from build123d import *

# Parameters (mm, degrees)
SKETCH1_R           = 23.8125
SKETCH1_R_2         = 20.6375
BOSS_EXTRUDE1_DEPTH = 8.89
BOSS_EXTRUDE2_START = -8.89
BOSS_EXTRUDE2_DEPTH = 8.89
FILLET1_R           = 25.4
CIRPATTERN1_DEPTH   = 8.89
SKETCH3_R           = 2.2225
CUT_EXTRUDE1_DEPTH  = 41.553113931
CIRPATTERN2_COUNT   = 6


# Read off the part's stored shape, not the designer's step: CirPattern1
with BuildPart() as part:
    # Sketch1 → Boss-Extrude1 (new body)
    with BuildSketch(Plane(origin=(0, 0, 0), x_dir=(1, 0, 0), z_dir=(0, 1, 0))):
        with Locations(Location((0, 0, 0), (0, 0, 270))):
            Circle(SKETCH1_R)
        with Locations(Location((0, 0, 0), (0, 0, 270))):
            Circle(SKETCH1_R_2, mode=Mode.SUBTRACT)
    extrude(amount=BOSS_EXTRUDE1_DEPTH)

    # Sketch2 → Boss-Extrude2 (add)
    with BuildSketch(Plane(origin=(0, 8.89, 0), x_dir=(1, 0, 0), z_dir=(0, 1, 0)).offset(BOSS_EXTRUDE2_START)):
        with BuildLine():
            ThreePointArc((-23.1267, 5.673702791), (-29.5275, 0), (-23.1267, -5.673702791))
            ThreePointArc((-23.1267, -5.673702791), (-23.8125, 0), (-23.1267, 5.673702791))
        make_face()
    extrude(amount=BOSS_EXTRUDE2_DEPTH)

    # Fillet1
    fillet1_edges = [part.edges().sort_by_distance(p)[0] for p in [
        (-23.1267, 4.445, -5.673702791),
        (-23.1267, 4.445, 5.673702791),
    ]]
    fillet(fillet1_edges, radius=FILLET1_R)

    # CirPattern1 outline → CirPattern1 (add)
    with BuildSketch(Plane(origin=(0, 0, 0), x_dir=(1, 0, 0), z_dir=(0, 1, 0))):
        with BuildLine():
            ThreePointArc((-20.530983871, -12.062912482), (-18.612348128, -16.535370154), (-17.581908256, -21.29165383))
            ThreePointArc((-17.581908256, -21.29165383), (-14.764885819, -25.570909171), (-9.650569001, -25.873242043))
            ThreePointArc((-9.650569001, -25.873242043), (-4.837563965, -24.35161844), (0.181296717, -23.811809838))
            ThreePointArc((0.181296717, -23.811809838), (-11.748897356, -20.712280588), (-20.530983871, -12.062912482))
        make_face()
        with BuildLine():
            ThreePointArc((-20.530983871, 12.062912482), (-11.90625, 20.622229928), (-0.181296717, 23.811809838))
            ThreePointArc((-0.181296717, 23.811809838), (-5.01387655, 24.38645138), (-9.648158978, 25.872206112))
            ThreePointArc((-9.648158978, 25.872206112), (-14.76375, 25.57156511), (-17.581908256, 21.29165383))
            ThreePointArc((-17.581908256, 21.29165383), (-18.612348128, 16.535370154), (-20.530983871, 12.062912482))
        make_face()
        with BuildLine():
            ThreePointArc((-0.181296717, 23.811809838), (11.748897356, 20.712280588), (20.530983871, 12.062912482))
            ThreePointArc((20.530983871, 12.062912482), (18.612348128, 16.535370154), (17.581908256, 21.29165383))
            ThreePointArc((17.581908256, 21.29165383), (14.764885819, 25.570909171), (9.650569001, 25.873242043))
            ThreePointArc((9.650569001, 25.873242043), (4.837563965, 24.35161844), (-0.181296717, 23.811809838))
        make_face()
        with BuildLine():
            ThreePointArc((20.530983871, 12.062912482), (23.811809838, 0.181296717), (20.712280588, -11.748897356))
            ThreePointArc((20.712280588, -11.748897356), (23.626224678, -7.851081226), (27.230067234, -4.580552281))
            ThreePointArc((27.230067234, -4.580552281), (29.527499849, -0.001311618), (27.232169388, 4.578983105))
            ThreePointArc((27.232169388, 4.578983105), (23.507902174, 7.986355934), (20.530983871, 12.062912482))
        make_face()
        with BuildLine():
            ThreePointArc((20.712280588, -11.748897356), (12.062912482, -20.530983871), (0.181296717, -23.811809838))
            ThreePointArc((0.181296717, -23.811809838), (5.01387655, -24.38645138), (9.648158978, -25.872206112))
            ThreePointArc((9.648158978, -25.872206112), (14.762614031, -25.572220789), (17.581600387, -21.294258937))
            ThreePointArc((17.581600387, -21.294258937), (18.67033821, -16.365262506), (20.712280588, -11.748897356))
        make_face()
    extrude(amount=CIRPATTERN1_DEPTH)

    # Sketch3 → Cut-Extrude1 (cut, symmetric)
    with BuildSketch(Plane(origin=(0, 8.89, 0), x_dir=(1, 0, 0), z_dir=(0, 1, 0))):
        with Locations(Location((-25.0825, 0, 0), (0, 0, 270))):
            Circle(SKETCH3_R)
    cut_extrude1 = extrude(amount=CUT_EXTRUDE1_DEPTH, both=True, mode=Mode.SUBTRACT)

    # CirPattern2: Cut-Extrude1 ×6 about axis
    cirpattern2_axis = Axis((0, 0, 0), (0, 1, 0))
    for i in range(1, CIRPATTERN2_COUNT):
        add(cut_extrude1.rotate(cirpattern2_axis, i * 360 / CIRPATTERN2_COUNT), mode=Mode.SUBTRACT)


solid = part.part
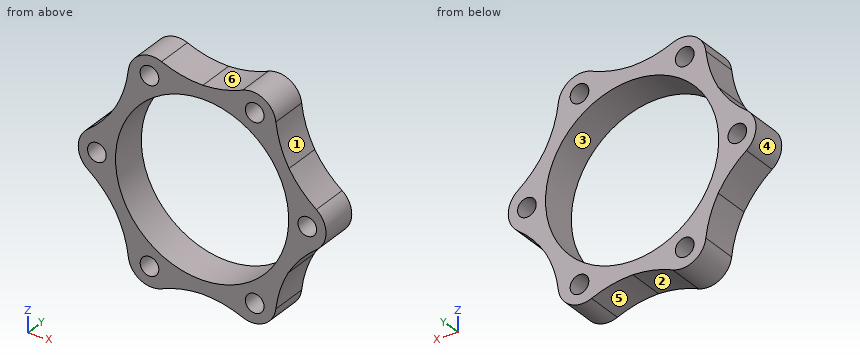
Read the model definition and answer for the solid it produces. Units are mm, in the model's axes. Face numbers are marked on the shaded views. A direction names the side the tool comes from. Round coordinates to 2 decimals unless told otherwise and drop trailing zeros. Write each loop counter-clockwise with the first axis right and the second up, starting at its lowest first coordinate (ties: lowest second). Pieces come first, ordered by that corner, then holes.
Q1. Find section D-D on x = 8. Determine the outline of the cut face in (y, z), and give its area (3 significant figures).
Values:
outline: (0, -25.23) - (8.89, -25.23) - (8.89, -19.02) - (0, -19.02) - close; (0, 19.02) - (8.89, 19.02) - (8.89, 25.23) - (0, 25.23) - close
area: 110 mm2
Q2. Find section A-A on z = 0. Determine the outline of the cut face in (x, y) (1 decimal).
Values:
outline: (-29.5, 0) - (-27.3, 0) - (-27.3, 8.9) - (-29.5, 8.9) - close; (-22.9, 0) - (-20.6, 0) - (-20.6, 8.9) - (-22.9, 8.9) - close; (20.6, 0) - (22.9, 0) - (22.9, 8.9) - (20.6, 8.9) - close; (27.3, 0) - (29.5, 0) - (29.5, 8.9) - (27.3, 8.9) - close
Q3. Straight lines are drawn through the part: line 1 (X direction, y = 5.5, z = 0) (1 decimal); line 2 (Z direction, x = -14, y = 2.5); line 3 (X direction, y = 2.5, z = -1). For each, find the intervals that lie inside material, in ascending order.
Values:
line 1: x = -29.5 to -27.3, -22.9 to -20.6, 20.6 to 22.9, 27.3 to 29.5
line 2: z = -25.94 to -23.4, -20.05 to -15.16, 15.16 to 20.05, 23.4 to 25.94
line 3: x = -29.44 to -27.07, -23.1 to -20.61, 20.61 to 23.1, 27.07 to 29.44
Q4. Find section B-B on x = -9. Determine the outline of the cut face in (y, z).
Values:
outline: (0, -25.6) - (8.89, -25.6) - (8.89, -18.57) - (0, -18.57) - close; (0, 18.57) - (8.89, 18.57) - (8.89, 25.6) - (0, 25.6) - close
Q5. The mould has two halves that part along Z. Classify the marked faces 1, 2 and 3: released by +Z, released by -Z, zero draft, split by the parting line, or undercut.
Values:
face 1: released by +Z
face 2: released by -Z
face 3: undercut
Q6. A tool of negligible diameter and unlimited length cuts with its end or side. For the marked faces 4, 5 and 6, from which of +Z, -Z, +X, -X, +Y, -Y can it reach the whole face along a straight path? Write none if from no direction.
Values:
face 4: -X, +Y, -Y
face 5: -Z, +Y, -Y
face 6: +Z, +Y, -Y
Q7. Find section C-C on z = -22. Determine the outline of the cut face in (x, y).
Values:
outline: (-17.45, 0) - (-14.75, 0) - (-14.75, 8.89) - (-17.45, 8.89) - close; (-10.34, 0) - (10.34, 0) - (10.34, 8.89) - (-10.34, 8.89) - close; (14.75, 0) - (17.45, 0) - (17.45, 8.89) - (14.75, 8.89) - close
Q8. Flat-ended cylindrical pins translate along their axes: P1, Ø3.5, axis at x = -25.08, z = 0, coming from the -Y side; P2, Ø7, axis at x = -12.54, z = -21.72, coming from the -Y side; P3, Ø4, axis at y = 4, z = -5.5, coming from the -X side; P4, Ø2, axis at y = 5, z = -9.5, coming from the +X side. Find the tip coordinate at first contact, or state that the pin passes through.
Values:
P1: passes through
P2: stops at y = 0
P3: stops at x = -28.33
P4: stops at x = 23.06
